Job drawing, mm, ordinate dimensions from the low corner. One solid piece. Round coordinates to 2 decimals unless told otherwise and drop trailing zeros. Loops run counter-clockwise (first coordinate to the right, second up) from the corner with the lowest first, then second, coordinate; pieces in that order, holes last.
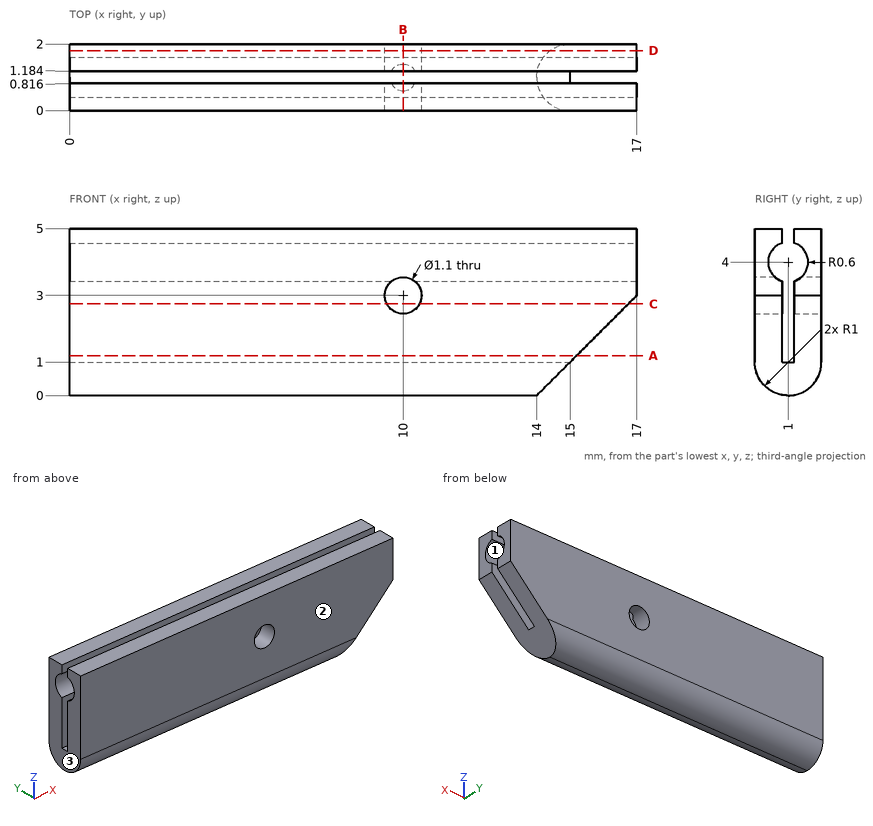
1) Wall check: line 1 along Y through (x, z) = (7.5, 2.5); line 2 along Y through (x, z) = (7, 4.05); line 3 along X through (y, z) = (0.7, 3.35) (1 decimal). Give the ranges that are in metal, low to high.
Values:
line 1: y = 0 to 0.82, 1.18 to 2
line 2: y = 0 to 0.4, 1.6 to 2
line 3: x = 0 to 9.6, 10.4 to 17
2) Slice it at B-B, the plane x = 10. Give the number of separate pieces and of enclosed holes in the cut face.
Values:
separate pieces: 3
enclosed holes: 0
3) Drop a flat-ended pin along its axis: pin 1 Ø0.7 at (x, z) = (10, 3) entering from +Y. Give the stop position or say it passes through.
Values:
pin 1: passes through
4) Mould opens along Y. For the marked faces 1, 2 and 3 say: released by +Y, released by -Y, zero draft, split by the parting line, or undercut.
Values:
face 1: undercut
face 2: released by -Y
face 3: zero draft
5) Slice it at C-C, the plane z = 2.75. Give the cut face in (x, y).
Values:
outline: (0, 0) - (9.51, 0) - (9.51, 0.82) - (0, 0.82) - close; (0, 1.18) - (9.51, 1.18) - (9.51, 2) - (0, 2) - close; (10.49, 0) - (16.75, 0) - (16.75, 0.82) - (10.49, 0.82) - close; (10.49, 1.18) - (16.75, 1.18) - (16.75, 2) - (10.49, 2) - close
6) Slice it at A-A, the plane z = 1.2. Give the cut face in (x, y).
Values:
outline: (0, 0) - (15.2, 0) - (15.2, 0.82) - (0, 0.82) - close; (0, 1.18) - (15.2, 1.18) - (15.2, 2) - (0, 2) - close
7) Slice it at D-D, the plane y = 1.8. Give the cut face in (x, z).
Values:
outline: (0, 0.4) - (14.4, 0.4) - (17, 3) - (17, 5) - (0, 5) - close; hole circle Ø1.1 at (10, 3)
